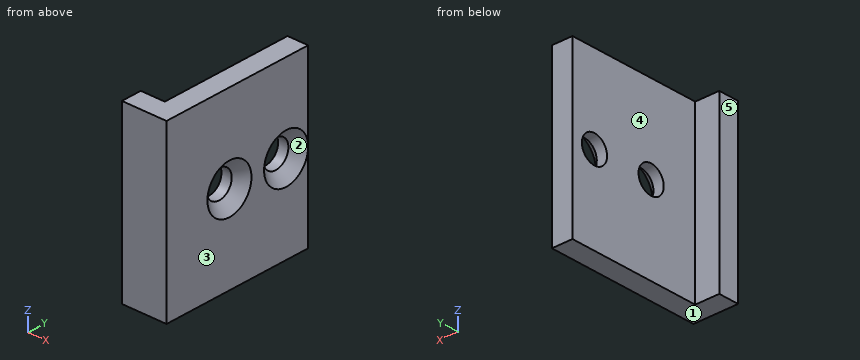
from build123d import *

# Parameters (mm, degrees)
BOSS_EXTRUDE1_DEPTH   = 25
F_1_0MM_DOWEL_HOLE1_D = 8
CHAMFER1_SIZE         = 3


with BuildPart() as part:
    # Sketch1 → Boss-Extrude1 (new, symmetric)
    with BuildSketch(Plane.XY):
        Polygon((-59.365603585, 18.386149477), (-59.365603585, 63.386149477), (-65.365603585, 63.386149477), (-65.365603585, 24.386149477), (-72.365603585, 24.386149477), (-72.365603585, 18.386149477), align=None)
    extrude(amount=BOSS_EXTRUDE1_DEPTH, both=True)

    # Ø1.0mm Dowel Hole1 (through all)
    with Locations(Plane(origin=(-59.365603585, 0, 0), x_dir=(0, 0, -1), z_dir=(1, 0, 0))):
        with Locations((0, 56.386149477), (0, 38.386149477)):
            Hole(F_1_0MM_DOWEL_HOLE1_D / 2)

    # Chamfer1
    chamfer1_edges = [part.edges().sort_by_distance(p)[0] for p in [
        (-59.365603585, 38.386149477, -4),
        (-59.365603585, 56.386149477, -4),
    ]]
    chamfer(chamfer1_edges, length=CHAMFER1_SIZE - 0.0001)  # a hair under: the kernel refuses the full size


solid = part.part
Can you work these out from the model? Positions are in its coordinate system, mm. Face numbers are marked on the shaded views. A direction names the side the tool comes from. Coordinates: 2 decimals unless noted, no trailing zeros. Loops run counter-clockwise (first coordinate to the right, second up) from the corner with the lowest first, then second, coordinate; pieces in that order, holes last. Notation, with made-up numbers: (-28, 33.25) - (-23, 33.25) arc R25 ccw to (-23, 61.25) - close; hole circle Ø10 at (-25.5, -2.5). An arc over 180 degrees is marked (long way). Put each result on its own line as item: value. Start each with the question number.
Item 1: Suppose I cut it at C-C (z = 18). Please give me the cut outline in (x, y).
Item 2: Which directions (+Z, -Z, +X, -X, +Y, -Y) give clear straight access to the entire face, cutting with the end or side of a thin tool? Please do the marked faces 4 and 5.
Item 3: Suppose I cut it at A-A (z = 0). State how many separate pieces and enclosed holes the cut face has, and give its area (3 significant figures).
Item 4: For pin 1 (6 mm diameter, centred on y = 58.5, z = 5.5, fed in from +X); pin 2 (19.5 mm diameter, centred on y = 38.5, z = -1, fed in from -X); pin 3 (7 mm diameter, centred on y = 38.39, z = 0, fed in from +X), each with a flat end and sliding along its axis, tell me the tip position at first contact or that it passes through.
Item 5: Suppose I cut it at D-D (x = -61.25). Please give me the cut outline in (y, z), and give its area (3 significant figures).
Item 6: Suppose I cut it at B-B (x = -64.25). Please give me the cut outline in (y, z).
Item 7: If I drill on line 1 along Y through (x, z) = (-64.2, 0); line 2 along X through (y, z) = (35.5, -13); line 3 along Z through (x, y) = (-63, 37), over which ranges is the centre line in solid material (lowest first)?
Item 8: If we mould it in two halves opening along Z, with no side actions, what happens to the marked faces 1, 2 and 3? For each: +Z half, -Z half, draft (parallel to the pull), parting line (faces both ways), or undercut.
Here are the results:
1. outline: (-72.37, 18.39) - (-59.37, 18.39) - (-59.37, 63.39) - (-65.37, 63.39) - (-65.37, 24.39) - (-72.37, 24.39) - close
2. face 4: +Z, -Z, -X, +Y
2. face 5: +Z, -Z, -X, +Y, -Y
3. separate pieces: 3
3. enclosed holes: 0
3. area: 198 mm²
4. pin 1: x = -59.37
4. pin 2: x = -65.37
4. pin 3: through
5. outline: (18.39, -25) - (63.39, -25) - (63.39, 25) - (18.39, 25) - close; hole circle Ø10.23 at (38.39, 0); hole circle Ø10.23 at (56.39, 0)
5. area: 2,090 mm²
6. outline: (18.39, -25) - (63.39, -25) - (63.39, 25) - (18.39, 25) - close; hole circle Ø8 at (38.39, 0); hole circle Ø8 at (56.39, 0)
7. line 1: 18.39 to 34.39, 42.39 to 52.39, 60.39 to 63.39
7. line 2: -65.37 to -59.37
7. line 3: -25 to -3.75, 3.75 to 25
8. face 1: -Z half
8. face 2: undercut
8. face 3: draft
